```python
from build123d import *

# Parameters (mm, degrees)
SKETCH2_W           = 32
SKETCH2_H           = 69.12
BOSS_EXTRUDE1_DEPTH = 18.34
CUT_EXTRUDE1_DEPTH  = 29
SKETCH4_R           = 2.305
BOSS_EXTRUDE3_DEPTH = 6


with BuildPart() as part:
    # Sketch2 → Boss-Extrude1 (new body)
    with BuildSketch(Plane(origin=(0, 0, 0), x_dir=(1, 0, 0), z_dir=(0, 1, 0))):
        Rectangle(SKETCH2_W, SKETCH2_H)
    extrude(amount=BOSS_EXTRUDE1_DEPTH)

    # Sketch3 → Cut-Extrude1 (cut)
    with BuildSketch(Plane(origin=(16, 0, 0), x_dir=(0, 0, -1), z_dir=(1, 0, 0))):
        Polygon((-23.6, 15.34), (10.4, 15.34), (10.4, 3), (-21.6, 3), (-21.6, 0), (-23.6, 0), (-23.6, 3), align=None)
    extrude(amount=-CUT_EXTRUDE1_DEPTH, mode=Mode.SUBTRACT)

    # Sketch4 → Boss-Extrude3 (add)
    with BuildSketch(Plane.ZY.offset(16)):
        with Locations(Location((0, 9.17, 0), (0, 0, 180))):
            Circle(SKETCH4_R)
    extrude(amount=BOSS_EXTRUDE3_DEPTH)


solid = part.part
```
The model under review builds one solid part; all positions refer to its coordinate system, in mm. A direction names the side the tool comes from. Round coordinates to 2 decimals unless told otherwise and drop trailing zeros. Loops run counter-clockwise (first coordinate to the right, second up) from the corner with the lowest first, then second, coordinate; pieces in that order, holes last. Notation, with made-up numbers: (56.25, -33) - (111.25, -33) arc R20 ccw to (111.25, -28) - close; hole circle Ø4 at (51, 50). An arc over 180 degrees is marked (long way). Use a Markdown table: item, result. Add a question column.
Q1. Add section B-B (y = 4.5). State the section outline as (x, z) points.
Q2. Add section A-A (z = 0). State the section outline as (x, y) points (3 decimals), plus the area to 3 significant figures.
Q3. Add section C-C (x = 8.5). State the section outline as (y, z) points, plus the area to 3 significant figures.
Q4. Insertion check: pin 1 Ø1.5 at (y, z) = (3.5, -8.5) entering from +X; pin 2 Ø7.5 at (y, z) = (7.5, 13.5) entering from +X. Each pin has a flat end and moves straight along its axis. Give the tip position at first contact, or say it passes through.
Q5. Add section D-D (y = 9.17). State the section outline as (x, z) points (3 decimals), plus the area to 3 significant figures.
Q6. For probe 1 along Y at (x, z) = (0.5, -9.5); probe 2 along Z at (x, y) = (5, 3.25); probe 3 along X at (y, z) = (6.75, 0), list the stretches that pass through material, from the lowest coordinate up.
Q7. The part is to be moulded in two halves that separate along Z. For faces 1 (the face through (-16, 13, 0)), 2 (the face through (2, 9, -10.4)), 3 (the face through (2, 2, 21.6)), 4 (the face through (0, 9, 34.56)), say which applies: pulls with the +Z half, pulls with the -Z half, needs draft (parallel to the pull), parting line crosses it, or undercut.
Q8. Machinability: for faces 5 (the face through (-18.958, 9.069, 2.303)), 6 (the face through (2, 8, 23.6)), 7 (the face through (2, 15.34, 7)), which of the approach directions +Z, -Z, +X, -X, +Y, -Y give a long, thin tool a straight path to every point of the face, cutting with its end or side? Answer none if there is none.
Worked answers:
| question | item | result |
|---|---|---|
| 1 | outline | (-16, -34.56) - (16, -34.56) - (16, -10.4) - (-13, -10.4) - (-13, 23.6) - (16, 23.6) - (16, 34.56) - (-16, 34.56) - close |
| 2 | outline | (-22, 6.865) - (-16, 6.865) - (-16, 0) - (16, 0) - (16, 3) - (-13, 3) - (-13, 15.34) - (16, 15.34) - (16, 18.34) - (-16, 18.34) - (-16, 11.475) - (-22, 11.475) - close |
| 2 | area | 257 mm² |
| 3 | outline | (0, -34.56) - (18.34, -34.56) - (18.34, 34.56) - (0, 34.56) - (0, 23.6) - (15.34, 23.6) - (15.34, -10.4) - (3, -10.4) - (3, 21.6) - (0, 21.6) - close |
| 3 | area | 842 mm² |
| 4 | pin 1 | x = 16 |
| 4 | pin 2 | x = -13 |
| 5 | outline | (-22, -2.305) - (-16, -2.305) - (-16, -34.56) - (16, -34.56) - (16, -10.4) - (-13, -10.4) - (-13, 23.6) - (16, 23.6) - (16, 34.56) - (-16, 34.56) - (-16, 2.305) - (-22, 2.305) - close |
| 5 | area | 1,250 mm² |
| 6 | probe 1 | 0 to 3, 15.34 to 18.34 |
| 6 | probe 2 | -34.56 to -10.4, 23.6 to 34.56 |
| 6 | probe 3 | -16 to -13 |
| 7 | face 1 | needs draft |
| 7 | face 2 | undercut |
| 7 | face 3 | undercut |
| 7 | face 4 | pulls with the +Z half |
| 8 | face 5 | -X |
| 8 | face 6 | +X, -Y |
| 8 | face 7 | +X |
